```python
from build123d import *

# Parameters (mm, degrees)
F0_R     = 4.35
F1_DEPTH = 50
F3_DEPTH = 15


with BuildPart() as f1:
    # F0 (on Front) → F1 (new body)
    with BuildSketch(Plane.XZ):
        with BuildLine():
            add(Edge.make_bspline(
                [(12.9, 20), (13.075, 11.616667), (13.425, 0), (13.075, -11.616667), (12.9, -20)],
                knots=[0, 0, 0, 0, 20.003062, 40.006125, 40.006125, 40.006125, 40.006125], degree=3))
            ThreePointArc((12.9, 20), (0, 32.9), (-12.9, 20))
            add(Edge.make_bspline(
                [(-12.9, 20), (-13.075, 11.616667), (-13.425, 0), (-13.075, -11.616667), (-12.9, -20)],
                knots=[0, 0, 0, 0, 20.003062, 40.006125, 40.006125, 40.006125, 40.006125], degree=3))
            ThreePointArc((-12.9, -20), (0, -32.9), (12.9, -20))
        make_face()
        with Locations((0, -20)):
            Circle(F0_R, mode=Mode.SUBTRACT)
        with Locations((0, 20)):
            Circle(F0_R, mode=Mode.SUBTRACT)
    extrude(amount=-F1_DEPTH)

    # F2 (on Right) → F3 (cut, symmetric)
    with BuildSketch(Plane.YZ):
        with BuildLine():
            Line((0, 14.4), (0, -14.4))
            ThreePointArc((0, -14.4), (14.4, 0), (0, 14.4))
        make_face()
        with BuildLine():
            Line((50, -32.9), (50, 32.9))
            Line((50, 32.9), (30, 32.9))
            Line((30, 32.9), (30, 14.4))
            ThreePointArc((30, 14.4), (44.4, 0), (30, -14.4))
            Line((30, -14.4), (30, -32.9))
            Line((30, -32.9), (50, -32.9))
        make_face()
    extrude(amount=F3_DEPTH, both=True, mode=Mode.SUBTRACT)


solid = f1.part
```
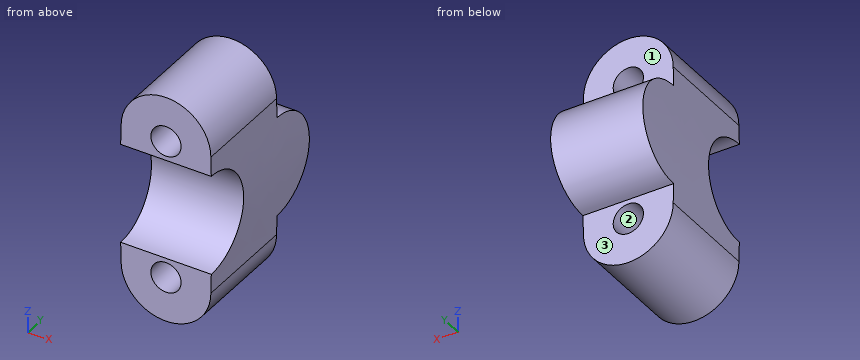
For this review, take the finished solid that the model builds, in its own axes (mm). Face numbers are marked on the shaded views. A direction names the side the tool comes from. Round coordinates to 2 decimals unless told otherwise and drop trailing zeros. Write each loop counter-clockwise with the first axis right and the second up, starting at its lowest first coordinate (ties: lowest second). Pieces come first, ordered by that corner, then holes. Notation, with made-up numbers: (86, 45) - (137, 45) arc R20 ccw to (137, 56) - close; hole circle Ø8 at (-6.75, 35.5). An arc over 180 degrees is marked (long way). Answer as CSV lines item,"result". Start each with the question number.
(1) For pin 1 (12 mm diameter, centred on y = 32, z = -12.5, fed in from -X); pin 2 (4 mm diameter, centred on y = 24.5, z = -13, fed in from -X); pin 3 (15 mm diameter, centred on x = 3.5, z = -26.5, fed in from +Y); pin 4 (8 mm diameter, centred on x = 0, z = 20, fed in from +Y), all flat-tipped, find the tip position at first contact; note any pin that passes through.
(2) Add section C-C, the plane x = -10. State the section outline as (y, z) points, plus the area to 3 significant figures.
(3) For line 1 (Z direction, x = 0, y = 18.5); line 2 (Z direction, x = -3, y = 16.5); line 3 (Z direction, x = -3.5, y = 6.5), list the stretches that pass through material, from the lowest coordinate up.
(4) Add section B-B, the plane y = 5. State how many separate pieces and enclosed holes the cut face has, plus the area to 3 significant figures.
(5) Add section A-A, the plane x = 0. State the section outline as (y, z) points.
(6) Machinability: for the marked faces 1, 2 and 3, which of the approach directions +Z, -Z, +X, -X, +Y, -Y give a long, thin tool a straight path to every point of the face, cutting with its end or side? Answer none if there is none.
From the geometry:
1,pin 1,"stops at x = -13.19"
1,pin 2,"stops at x = -13.1"
1,pin 3,"stops at y = 30"
1,pin 4,"passes through"
2,outline,"(0, -28.15) - (30, -28.15) - (30, -14.4) arc R14.4 ccw to (30, 14.4) - (30, 28.15) - (0, 28.15) - (0, 14.4) arc R14.4 cw to (0, -14.4) - close"
2,area,"1,690 mm²"
3,line 1,"z = -32.9 to -24.35, -15.65 to 15.65, 24.35 to 32.9"
3,line 2,"z = -32.55 to -23.15, -16.85 to 16.85, 23.15 to 32.55"
3,line 3,"z = -32.42 to -22.58, -17.42 to -12.85, 12.85 to 17.42, 22.58 to 32.42"
4,separate pieces,"2"
4,enclosed holes,"2"
4,area,"741 mm²"
5,outline,"(0, -32.9) - (30, -32.9) - (30, -24.35) - (0, -24.35) - close; (0, -15.65) - (30, -15.65) - (30, -14.4) arc R14.4 ccw to (30, 14.4) - (30, 15.65) - (0, 15.65) - (0, 14.4) arc R14.4 cw to (0, -14.4) - close; (0, 24.35) - (30, 24.35) - (30, 32.9) - (0, 32.9) - close"
6,face 1,"+Z, +X, -X, +Y"
6,face 2,"+Y, -Y"
6,face 3,"-Z, +X, -X, +Y"
